Here's how the part is built. I have some questions about the finished solid (model axes, mm). A direction names the side the tool comes from. Give positions to 0.01 mm unless a question says otherwise; leave off trailing zeros. Loops run counter-clockwise (first coordinate to the right, second up) from the corner with the lowest first, then second, coordinate; pieces in that order, holes last.
Q1. Suppose I cut it at A-A (z = 6). List the corners of the cut face in (x, y) for me, and give its area (3 significant figures).
Q2. Thinking about a two-plate mould opening in X: for faces 3 (the face through (27, -7, 1)), 4 (the face through (27, -2, 38)), 5 (the face through (45.14, -1.52, 37.1)), 6 (the face through (0.86, -3.55, 0.9)), which applies, pulls with the +X half, pulls with the -X half, needs draft (parallel to the pull), parting line crosses it, or undercut?
Q3. Suppose I cut it at D-D (x = 9.5). List the corners of the cut face in (y, z) for me, and give its area (3 significant figures).
Q4. For faces 1 (the face through (27, 0, 9)), 2 (the face through (52, -5, 25)), which set-ups out of +Z, -Z, +X, -X, +Y, -Y let a thin tool reach every point of the face, with its end or its side?
Q5. I need wall thicknesses on probe 1 along Z at (x, y) = (27.5, -6); probe 2 along Z at (x, y) = (25, -2.5); probe 3 along Z at (x, y) = (9, -2.25). Which ranges of each line are inside material? Lowest first, please.
Q6. Suppose I cut it at B-B (y = -2.25). List the corners of the cut face in (x, z) for me.
Q7. I'm going to push flat-ended pins straight in: P1, Ø2, axis at x = 9, z = 44, coming from the +Y side; P2, Ø14, axis at x = 23.5, z = 17.5, coming from the -Y side. Where does each tip first touch, or does it pass through?
Q8. Suppose I cut it at C-C (z = 22.5). List the corners of the cut face in (x, y) for me.
```python
from build123d import *

# Parameters (mm, degrees)
F0_W     = 54
F0_H     = 50
F1_DEPTH = 7
F3_D     = 3.4
F5_DEPTH = 25
F7_DEPTH = 4
F8_R     = 3


with BuildPart() as f1:
    # F0 (on Front) → F1 (new body)
    with BuildSketch(Plane.XZ):
        with Locations((27, 25)):
            Rectangle(F0_W, F0_H)
    extrude(amount=F1_DEPTH)

    # F3 (through all)
    with Locations(Plane.XZ.offset(7)):
        with Locations((9, 44), (45, 44), (9, 6), (45, 6)):
            Hole(F3_D / 2)

    # F4 (on face) → F5 (cut)
    with BuildSketch(Plane.XZ.offset(7)):
        with BuildLine():
            Line((43, 38), (11, 38))
            ThreePointArc((11, 38), (8.8786796564, 37.1213203436), (8, 35))
            Line((8, 35), (8, 15))
            ThreePointArc((8, 15), (8.8786796564, 12.8786796564), (11, 12))
            Line((11, 12), (43, 12))
            ThreePointArc((43, 12), (45.1213203436, 12.8786796564), (46, 15))
            Line((46, 15), (46, 35))
            ThreePointArc((46, 35), (45.1213203436, 37.1213203436), (43, 38))
        make_face()
    extrude(amount=-F5_DEPTH, mode=Mode.SUBTRACT)

    # F6 (on face) → F7 (cut)
    with BuildSketch(Plane.XZ.offset(7)):
        with BuildLine():
            Line((4.1184528013, 47.9964891519), (3.881241658, 47.9964710006))
            ThreePointArc((3.881241658, 47.9964710006), (2.5444044717, 47.3715836314), (2, 46))
            ThreePointArc((2, 46), (4, 44), (6, 46))
            ThreePointArc((6, 46), (5.4554905707, 47.3716950093), (4.1184528013, 47.9964891519))
        make_face()
        with BuildLine():
            ThreePointArc((4.1184528013, 47.9964891519), (3.9998469603, 47.9999999941), (3.881241658, 47.9964710006))
            Line((3.881241658, 47.9964710006), (4.1184528013, 47.9964891519))
        make_face()
        with BuildLine():
            ThreePointArc((6, 46), (4, 44), (2, 46))
            Line((2, 46), (2, 4))
            ThreePointArc((2, 4), (4, 6), (6, 4))
            ThreePointArc((6, 4), (5.4142135624, 2.5857864376), (4, 2))
            Line((4, 2), (50, 2))
            ThreePointArc((50, 2), (48.5857864376, 5.4142135624), (52, 4))
            Line((52, 4), (52, 46))
            ThreePointArc((52, 46), (48.5857864376, 44.5857864376), (50, 48))
            Line((50, 48), (4.1184528013, 47.9964891519))
            ThreePointArc((4.1184528013, 47.9964891519), (5.4554905707, 47.3716950093), (6, 46))
        make_face()
        with BuildLine():
            Line((4, 2), (2, 4))
            ThreePointArc((2, 4), (2.5857864376, 2.5857864376), (4, 2))
        make_face()
        with BuildLine():
            ThreePointArc((6, 4), (4, 6), (2, 4))
            Line((2, 4), (4, 2))
            ThreePointArc((4, 2), (5.4142135624, 2.5857864376), (6, 4))
        make_face()
        with BuildLine():
            Line((52, 46), (50, 48))
            ThreePointArc((50, 48), (48.5857864376, 44.5857864376), (52, 46))
        make_face()
        with BuildLine():
            ThreePointArc((52, 46), (51.4142135624, 47.4142135624), (50, 48))
            Line((50, 48), (52, 46))
        make_face()
        with BuildLine():
            Line((52, 4), (50, 2))
            ThreePointArc((50, 2), (51.4142135624, 2.5857864376), (52, 4))
        make_face()
        with BuildLine():
            ThreePointArc((52, 4), (48.5857864376, 5.4142135624), (50, 2))
            Line((50, 2), (52, 4))
        make_face()
    extrude(amount=-F7_DEPTH, mode=Mode.SUBTRACT)

    # F8
    f8_edges = [f1.edges().sort_by_distance(p)[0] for p in [
        (54, -3.5, 50),
        (54, -3.5, 0),
        (0, -3.5, 0),
        (0, -3.5, 50),
    ]]
    fillet(f8_edges, radius=F8_R)


solid = f1.part
```
Solutions:
1. outline: (0, -7) - (2, -7) - (2, -3) - (7.3, -3) - (7.3, 0) - (0, 0) - close; (10.7, -3) - (43.3, -3) - (43.3, 0) - (10.7, 0) - close; (46.7, -3) - (52, -3) - (52, -7) - (54, -7) - (54, 0) - (46.7, 0) - close
1. area: 158 mm2
2. face 3: needs draft
2. face 4: undercut
2. face 5: undercut
2. face 6: pulls with the -X half
3. outline: (-7, 0) - (0, 0) - (0, 4.38) - (-3, 4.38) - (-3, 2) - (-7, 2) - close; (-7, 48) - (-3, 48) - (-3, 45.62) - (0, 45.62) - (0, 50) - (-7, 50) - close; (-3, 7.62) - (0, 7.62) - (0, 12.4) - (-3, 12.4) - close; (-3, 37.6) - (0, 37.6) - (0, 42.38) - (-3, 42.38) - close
3. area: 70.9 mm2
4. face 1: +Z, -Z, +X, -X, +Y
4. face 2: -Y
5. probe 1: z = 0 to 2, 48 to 50
5. probe 2: z = 0 to 12, 38 to 50
5. probe 3: z = 0 to 4.3, 7.7 to 12.76, 37.24 to 42.3, 45.7 to 50
6. outline: (0, 3) arc R3 ccw to (3, 0) - (51, 0) arc R3 ccw to (54, 3) - (54, 47) arc R3 ccw to (51, 50) - (3, 50) arc R3 ccw to (0, 47) - close; hole circle Ø3.4 at (9, 6); hole circle Ø3.4 at (9, 44); hole (8, 15) arc R3 ccw to (11, 12) - (43, 12) arc R3 ccw to (46, 15) - (46, 35) arc R3 ccw to (43, 38) - (11, 38) arc R3 ccw to (8, 35) - close; hole circle Ø3.4 at (45, 6); hole circle Ø3.4 at (45, 44)
7. P1: passes through
7. P2: stops at y = -3
8. outline: (0, -7) - (2, -7) - (2, -3) - (8, -3) - (8, 0) - (0, 0) - close; (46, -3) - (52, -3) - (52, -7) - (54, -7) - (54, 0) - (46, 0) - close
